```python
from build123d import *

# Parameters (mm, degrees)
CROQUIS1_R              = 20
CROQUIS1_R_2            = 2.5
CROQUIS1_R_3            = 1.5
SALIENTE_EXTRUIR1_DEPTH = 5
CORTAR_EXTRUIR1_DEPTH   = 29.722813233
MATRIZC1_COUNT          = 18
CROQUIS3_R              = 5
CORTAR_EXTRUIR2_DEPTH   = 2.5


with BuildPart() as part:
    # Croquis1 → Saliente-Extruir1 (new body)
    with BuildSketch(Plane.XY):
        Circle(CROQUIS1_R)
        Circle(CROQUIS1_R_2, mode=Mode.SUBTRACT)
        with Locations((0, 10)):
            Circle(CROQUIS1_R_3, mode=Mode.SUBTRACT)
    extrude(amount=SALIENTE_EXTRUIR1_DEPTH)

    # Croquis2 → Cortar-Extruir1 (cut, through all)
    with BuildSketch(Plane.XY.offset(5)):
        with BuildLine():
            ThreePointArc((2.678584333, 19.819818011), (0, 20), (-2.678584333, 19.819818011))
            ThreePointArc((-2.678584333, 19.819818011), (-1.82600889, 18.733131722), (-1.522223543, 17.385731841))
            ThreePointArc((-1.522223543, 17.385731841), (-1.19593308, 16.445057276), (-0.5915417, 15.653827117))
            ThreePointArc((-0.5915417, 15.653827117), (0, 15.665), (0.5915417, 15.653827117))
            ThreePointArc((0.5915417, 15.653827117), (1.19593308, 16.445057276), (1.522223543, 17.385731841))
            ThreePointArc((1.522223543, 17.385731841), (1.82600889, 18.733131722), (2.678584333, 19.819818011))
        make_face()
    cortar_extruir1 = extrude(amount=-CORTAR_EXTRUIR1_DEPTH, mode=Mode.SUBTRACT)

    # MatrizC1: Cortar-Extruir1 ×18 about axis
    matrizc1_axis = Axis((0, 0, 0), (0, 0, 1))
    for i in range(1, MATRIZC1_COUNT):
        add(cortar_extruir1.rotate(matrizc1_axis, i * 360 / MATRIZC1_COUNT), mode=Mode.SUBTRACT)

    # Croquis3 → Cortar-Extruir2 (cut)
    with BuildSketch(Plane.XY.offset(5)):
        Circle(CROQUIS3_R)
    extrude(amount=-CORTAR_EXTRUIR2_DEPTH, mode=Mode.SUBTRACT)


solid = part.part
```
Input: part model. Units: mm. Frame: model coordinates. A direction names the side the tool comes from. Give positions to 0.01 mm unless a question says otherwise; leave off trailing zeros. Order: outer loops, then holes, each group sorted by start corner. A loop starts at its lowest first (then second) coordinate and runs counter-clockwise, first axis right, second up. Notation, with made-up numbers: (-23, 32) - (16, 32) arc R30 ccw to (16, 71) - close; hole circle Ø1 at (63, 23). An arc over 180 degrees is marked (long way). One line per item, written item: value.
1. Reachability of faces 1 (the face through (16.39, 1.682, 2.535)), 2 (the face through (13.64, -9.25, 2.54)), 3 (the face through (-15.3, 10.93, 2.54)), 4 (the face through (-1.834, 18.751, 2.535)), 5 (the face through (1.203, -16.457, 2.535)) from +Z, -Z, +X, -X, +Y, -Y: full face, straight path, thin tool, end or side. Return the list, or none.
Determined:
face 1: +Z, -Z
face 2: +Z, -Z, +X
face 3: +Z, -Z, -X
face 4: +Z, -Z, +Y
face 5: +Z, -Z, -Y
2. Cut plane C-C, the plane y = 9.5. Output: boundary loops of the cut face in (x, z), and give its area (3 significant figures).
Determined:
outline: (-13.81, 0) - (-1.41, 0) - (-1.41, 5) - (-13.81, 5) - close; (1.41, 0) - (13.81, 0) - (13.81, 5) - (1.41, 5) - close
area: 124 mm2
3. Cut plane B-B, the plane x = 0. Output: boundary loops of the cut face in (y, z) (3 decimals).
Determined:
outline: (-15.665, 0) - (-2.5, 0) - (-2.5, 2.5) - (-5, 2.5) - (-5, 5) - (-15.665, 5) - close; (2.5, 0) - (8.5, 0) - (8.5, 5) - (5, 5) - (5, 2.5) - (2.5, 2.5) - close; (11.5, 0) - (15.665, 0) - (15.665, 5) - (11.5, 5) - close
4. Draft query along Y for faces 6 (the face through (15.328, 12.847, 2.465)), 7 (the face through (-0.325, 8.536, 2.465)), 8 (the face through (9.99, -17.326, 2.465)). Return one class per face: released by +Y, released by -Y, zero draft, split by the parting line, or undercut.
Determined:
face 6: released by +Y
face 7: undercut
face 8: released by -Y
5. Line query: probe 1 along Y at (x, z) = (0, 1.25) (3 decimals); probe 2 along X at (y, z) = (17.5, 1.3); probe 3 along Y at (x, z) = (-10.5, 0.3). Output: solid intervals per line, ascending.
Determined:
probe 1: -15.665 to -2.5, 2.5 to 8.5, 11.5 to 15.665
probe 2: -9.68 to -8.83, -4.68 to -1.52, 1.52 to 4.68, 8.83 to 9.68
probe 3: -17.02 to -15.1, -11.63 to 11.63, 15.1 to 17.02
6. Cut plane D-D, the plane z = 1.8. Give the number of separate pieces and of enclosed holes in the cut face, and give its area (3 significant figures).
Determined:
separate pieces: 1
enclosed holes: 2
area: 981 mm2
7. Cut plane A-A, the plane y = 0. Output: boundary loops of the cut face in (x, z), and give its area (4 significant figures).
Determined:
outline: (-20, 0) - (-2.5, 0) - (-2.5, 2.5) - (-5, 2.5) - (-5, 5) - (-20, 5) - close; (2.5, 0) - (20, 0) - (20, 5) - (5, 5) - (5, 2.5) - (2.5, 2.5) - close
area: 162.5 mm2
8. Pin query (flat end, axial travel): pin 1 Ø1.5 at (x, z) = (7.5, 2.5) entering from +Y; pin 2 Ø1.5 at (y, z) = (14, 1.5) entering from -X; pin 3 Ø2 at (y, z) = (4.5, 2.5) entering from -X. Return the tip coordinate at first contact, or that it passes through.
Determined:
pin 1: y = 17.1
pin 2: x = -14.98
pin 3: x = -18.64
